Source: CAD feature listing. Evaluate the final solid. Frame: model axes, mm. A direction names the side the tool comes from. Give positions to 0.01 mm unless a question says otherwise; leave off trailing zeros. Order: outer loops, then holes, each group sorted by start corner. A loop starts at its lowest first (then second) coordinate and runs counter-clockwise, first axis right, second up.
from build123d import *

# Parameters (mm, degrees)
F0_W           = 60
F0_H           = 47
F1_DEPTH       = 5
F3_DEPTH       = 20
F4_W           = 60
F4_H           = 5
F5_DEPTH       = 28.5
F7_DEPTH       = 5
F9_DEPTH       = 8
F10_W          = 60
F10_H          = 5
F11_DEPTH      = 8
F12_R          = 2
F13_DEPTH      = 25
F15_DEPTH      = 2.5
F15_DEPTH_BACK = 2.5
F16_R          = 2
F17_DEPTH      = 75.501
F18_R          = 3.25
F19_DEPTH      = 28
F20_DEPTH      = 138


# Not quite as in the source:
# - an extrude ends at something that could not be found from the text; its depth is read off the source's solid
# - a pattern or mirror of a feature is missing from the dataset's text; its kind, count and spacing are read off the source's solid
# - a feature names something its author has since deleted; it is built from what else it names


with BuildPart() as f1:
    # F0 (on Top) → F1 (new body)
    with BuildSketch(Plane.XY):
        with Locations((0, -1.5)):
            Rectangle(F0_W, F0_H)
        with BuildLine():
            Line((-14, -14), (-14, -18))
            ThreePointArc((-14, -18), (-16, -20), (-18, -18))
            Line((-18, -18), (-18, -14))
            ThreePointArc((-18, -14), (-16, -12), (-14, -14))
        make_face(mode=Mode.SUBTRACT)
        with BuildLine():
            Line((18, -14), (18, -18))
            ThreePointArc((18, -18), (16, -20), (14, -18))
            Line((14, -18), (14, -14))
            ThreePointArc((14, -14), (16, -12), (18, -14))
        make_face(mode=Mode.SUBTRACT)
        with BuildLine():
            ThreePointArc((-14, 14), (-16, 12), (-18, 14))
            Line((-18, 14), (-18, 18))
            ThreePointArc((-18, 18), (-16, 20), (-14, 18))
            Line((-14, 18), (-14, 14))
        make_face(mode=Mode.SUBTRACT)
        with BuildLine():
            Line((-12, -2), (-12, 2))
            ThreePointArc((-12, 2), (0, 14), (12, 2))
            Line((12, 2), (12, -2))
            ThreePointArc((12, -2), (0, -14), (-12, -2))
        make_face(mode=Mode.SUBTRACT)
        with BuildLine():
            Line((14, 14), (14, 18))
            ThreePointArc((14, 18), (16, 20), (18, 18))
            Line((18, 18), (18, 14))
            ThreePointArc((18, 14), (16, 12), (14, 14))
        make_face(mode=Mode.SUBTRACT)
    extrude(amount=F1_DEPTH)

    # F2 (on face) → F3 (join)
    with BuildSketch(Plane.XY.offset(5)):
        with BuildLine():
            Line((30, 22), (-30, 22))
            Line((-30, 22), (-30, 17))
            Line((-30, 17), (-18, 17))
            Line((-18, 17), (-18, 18))
            ThreePointArc((-18, 18), (-16, 20), (-14, 18))
            Line((-14, 18), (-14, 17))
            Line((-14, 17), (14, 17))
            Line((14, 17), (14, 18))
            ThreePointArc((14, 18), (16, 20), (18, 18))
            Line((18, 18), (18, 17))
            Line((18, 17), (30, 17))
            Line((30, 17), (30, 22))
        make_face()
    extrude(amount=F3_DEPTH)

    # F4 (on face) → F5 (join)
    with BuildSketch(Plane(origin=(0, 22, 0), x_dir=(-1, 0, 0), z_dir=(0, 1, 0))):
        with Locations((0, 22.5)):
            Rectangle(F4_W, F4_H)
    extrude(amount=F5_DEPTH)

    # F6 (on face) → F7 (join)
    with BuildSketch(Plane(origin=(-30, 0, 0), x_dir=(0, -1, 0), z_dir=(-1, 0, 0))):
        Polygon((-22, 20), (-50.5, 20), (-22, 0), align=None)
        Polygon((25, 5), (-17, 25), (-17, 5), align=None)
    f7 = extrude(amount=-F7_DEPTH)

    # F7_copies: F7 across plane
    add(f7.mirror(Plane(origin=(0, 0, 0), x_dir=(0, 0, 1), z_dir=(1, 0, 0))))

    # F8 (on face) → F9 (join)
    with BuildSketch(Plane.XY.offset(25)):
        with BuildLine():
            Line((30, 22), (-30, 22))
            Line((-30, 22), (-30, 17))
            Line((-30, 17), (-25, 17))
            Line((-25, 17), (-18, 17))
            Line((-18, 17), (-18, 18))
            ThreePointArc((-18, 18), (-16, 20), (-14, 18))
            Line((-14, 18), (-14, 17))
            Line((-14, 17), (14, 17))
            Line((14, 17), (14, 18))
            ThreePointArc((14, 18), (16, 20), (18, 18))
            Line((18, 18), (18, 17))
            Line((18, 17), (25, 17))
            Line((25, 17), (30, 17))
            Line((30, 17), (30, 22))
        make_face()
    extrude(amount=F9_DEPTH)

    # F10 (on face) → F11 (join)
    with BuildSketch(Plane.XY.offset(25)):
        with Locations((0, 48)):
            Rectangle(F10_W, F10_H)
    extrude(amount=F11_DEPTH)

    # F12 (on face) → F13 (cut)
    with BuildSketch(Plane.XY.offset(25)):
        with Locations((14, 34)):
            Circle(F12_R)
        with Locations((-14, 34)):
            Circle(F12_R)
    extrude(amount=-F13_DEPTH, mode=Mode.SUBTRACT)

    # F14 (on Right) → F15 (join, two sides)
    with BuildSketch(Plane.YZ) as f15_sk:
        Polygon((22, 20), (22, 0), (50.5, 20), align=None)
    extrude(amount=F15_DEPTH)
    extrude(f15_sk.sketch, amount=-F15_DEPTH_BACK)

    # F16 (on face) → F17 (cut, through all)
    with BuildSketch(Plane(origin=(0, 50.5, 0), x_dir=(-1, 0, 0), z_dir=(0, 1, 0))):
        with Locations((-22, 28)):
            Circle(F16_R)
        with Locations((22, 28)):
            Circle(F16_R)
        with Locations((0, 28)):
            Circle(F16_R)
    extrude(amount=-F17_DEPTH, mode=Mode.SUBTRACT)

    # F18 (on face) → F19 (cut, through all)
    with BuildSketch(Plane.XY.offset(33)):
        with Locations((-16, 18)):
            Circle(F18_R)
        with Locations((16, 18)):
            Circle(F18_R)
    extrude(amount=-F19_DEPTH, mode=Mode.SUBTRACT)

    # F16 (on face) → F20 (cut, through all)
    with BuildSketch(Plane(origin=(0, 50.5, 0), x_dir=(-1, 0, 0), z_dir=(0, 1, 0))):
        with Locations((-22, 28)):
            Circle(F16_R)
        with Locations((22, 28)):
            Circle(F16_R)
        with Locations((0, 28)):
            Circle(F16_R)
    extrude(amount=F20_DEPTH, mode=Mode.SUBTRACT)


solid = f1.part
1) Pull-direction query (Y, two-part tool) for faces 1 (the face through (0, 48, 26)), 2 (the face through (-27.54, 36.45, 10.14)), 3 (the face through (16, 20, 2)); classes: +Y half, -Y half, draft (parallel to the pull), parting line (faces both ways), or undercut.
Checks:
face 1: draft
face 2: +Y half
face 3: undercut
2) Section query C-C on y = -17. Output: boundary loops of the cut face in (x, z), and give its area (3 significant figures).
Checks:
outline: (-30, 0) - (-18, 0) - (-18, 5) - (-25, 5) - (-25, 8.81) - (-30, 8.81) - close; (-14, 0) - (14, 0) - (14, 5) - (-14, 5) - close; (18, 0) - (30, 0) - (30, 8.81) - (25, 8.81) - (25, 5) - (18, 5) - close
area: 298 mm2
3) Ray query, L1, parallel to X at y = 14, z = 14; L2, parallel to Z at x = 22, y = 19.95; L3, parallel to X at y = 28, z = 6.5. Return the intervals inside material, ascending.
Checks:
L1: x = -30 to -25, 25 to 30
L2: z = 0 to 26, 30 to 33
L3: x = -30 to -25, -2.5 to 2.5, 25 to 30
4) Section query A-A on x = 0. Output: boundary loops of the cut face in (y, z), and give its area (4 significant figures).
Checks:
outline: (-25, 0) - (-14, 0) - (-14, 5) - (-25, 5) - close; (14, 0) - (22, 0) - (50.5, 20) - (50.5, 26) - (45.5, 26) - (45.5, 25) - (22, 25) - (22, 26) - (17, 26) - (17, 5) - (14, 5) - close; (17, 30) - (22, 30) - (22, 33) - (17, 33) - close; (45.5, 30) - (50.5, 30) - (50.5, 33) - (45.5, 33) - close
area: 662.5 mm2
5) Section query B-B on x = -22. Output: boundary loops of the cut face in (y, z).
Checks:
outline: (-25, 0) - (22, 0) - (22, 20) - (50.5, 20) - (50.5, 26) - (45.5, 26) - (45.5, 25) - (22, 25) - (22, 26) - (17, 26) - (17, 5) - (-25, 5) - close; (17, 30) - (22, 30) - (22, 33) - (17, 33) - close; (45.5, 30) - (50.5, 30) - (50.5, 33) - (45.5, 33) - close
6) First-contact query: pin 1 Ø6 at (x, y) = (-9.5, 3) entering from +Z; pin 2 Ø8 at (x, y) = (7.5, 30) entering from +Z; pin 3 Ø1.5 at (x, z) = (-10, 16) entering from +Y. Flat tips, straight axial feed; report the tip coordinate or a pass-through.
Checks:
pin 1: stops at z = 5
pin 2: stops at z = 25
pin 3: stops at y = 22
7) Section query D-D on z = 17. Output: boundary loops of the cut face in (x, y) (3 decimals), and give its area (3 significant figures).
Checks:
outline: (-30, 0.2) - (-25, 0.2) - (-25, 17) - (-19.092, 17) arc R3.25 cw (long way) to (-12.908, 17) - (12.908, 17) arc R3.25 cw (long way) to (19.092, 17) - (25, 17) - (25, 0.2) - (30, 0.2) - (30, 46.225) - (25, 46.225) - (25, 22) - (2.5, 22) - (2.5, 46.225) - (-2.5, 46.225) - (-2.5, 22) - (-25, 22) - (-25, 46.225) - (-30, 46.225) - close
area: 785 mm2
8) Reachability of faces 4 (the face through (0, 34, 25)), 5 (the face through (-25, 6, 11)), 6 (the face through (-11, 36, 20)), 7 (the face through (-15.91, 21.25, 19.2)), 8 (the face through (0, 14, 2)) from +Z, -Z, +X, -X, +Y, -Y: full face, straight path, thin tool, end or side. Return the list, or none.
Checks:
face 4: +Z, +X, -X
face 5: +Z, -Y
face 6: -Z, +Y
face 7: +Z
face 8: +Z, -Z
